```python
from build123d import *

# Parameters (mm, degrees)
F0_W     = 25
F0_H     = 31
F1_DEPTH = 86.3
F2_R     = 6.5
F3_DEPTH = 31.5
F5_DEPTH = 31.001


with BuildPart() as f1:
    # F0 (on Top) → F1 (new body)
    with BuildSketch(Plane.XY):
        Rectangle(F0_W, F0_H)
    extrude(amount=F1_DEPTH)

    # F2 (on Front) → F3 (cut, symmetric)
    with BuildSketch(Plane.XZ):
        with Locations((0, 58.577)):
            Circle(F2_R)
    extrude(amount=F3_DEPTH, both=True, mode=Mode.SUBTRACT)

    # F4 (on face) → F5 (cut, through all)
    with BuildSketch(Plane(origin=(0, 15.5, 0), x_dir=(-1, 0, 0), z_dir=(0, 1, 0))):
        Polygon((12.5, 0), (12.5, 86.3), (6, 0), align=None)
        Polygon((-6, 0), (-12.5, 86.3), (-12.5, 0), align=None)
    extrude(amount=-F5_DEPTH, mode=Mode.SUBTRACT)


solid = f1.part
```
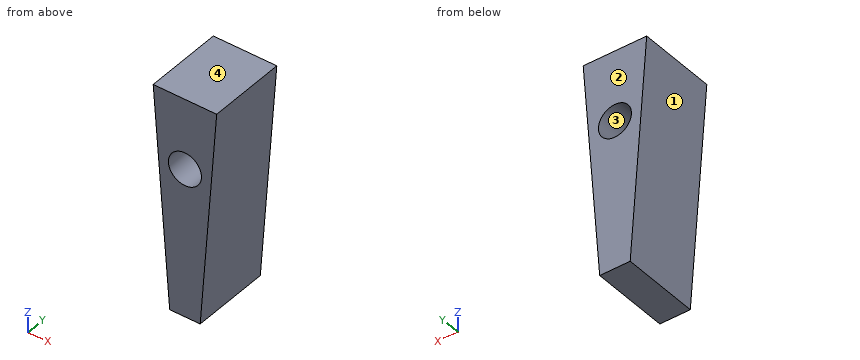
Check sheet for the modelled part. Datum: model origin and axes. Units: mm. Face numbers are marked on the shaded views. Round coordinates to 2 decimals unless told otherwise and drop trailing zeros. Order: outer loops, then holes, each group sorted by start corner. A loop starts at its lowest first (then second) coordinate and runs counter-clockwise, first axis right, second up.
1) Section check D-D (z = 31). Record the boundary of the cut face in (x, y), and give its area (3 significant figures).
2) Section check B-B (z = 60.5). Record the boundary of the cut face in (x, y).
3) Section check C-C (y = 1). Record the boundary of the cut face in (x, z).
4) Section check A-A (x = 0). Record the boundary of the cut face in (y, z).
5) Mould release check, pull along Z, two halves, no side actions. Record for the marked faces 1, 2, 3 and 4: +Z half, -Z half, draft (parallel to the pull), parting line (faces both ways), or undercut.
6) Scan lines: line 1 (Z direction, x = 0, y = -2); line 2 (X direction, y = 7.5, z = 63); line 3 (X direction, y = 7.5, z = 56.5). Record each from-to range of solid material in increasing order.
7) Go/stop test with flat-tipped pins: pin 1 Ø1 at (y, z) = (-12, 17) entering from -X; pin 2 Ø2 at (y, z) = (-9.5, 27) entering from +X; pin 3 Ø15 at (x, z) = (0, 58.577) entering from +Y; pin 4 Ø12 at (y, z) = (10.5, 63) entering from -X. Record where each tip stops, or that it passes through.
Result:
1. outline: (-8.33, -15.5) - (8.33, -15.5) - (8.33, 15.5) - (-8.33, 15.5) - close
1. area: 517 mm2
2. outline: (-10.56, -15.5) - (-6.21, -15.5) - (-6.21, 15.5) - (-10.56, 15.5) - close; (6.21, -15.5) - (10.56, -15.5) - (10.56, 15.5) - (6.21, 15.5) - close
3. outline: (-12.5, 86.3) - (-6, 0) - (6, 0) - (12.5, 86.3) - close; hole circle Ø13 at (0, 58.58)
4. outline: (-15.5, 0) - (15.5, 0) - (15.5, 52.08) - (-15.5, 52.08) - close; (-15.5, 65.08) - (15.5, 65.08) - (15.5, 86.3) - (-15.5, 86.3) - close
5. face 1: -Z half
5. face 2: draft
5. face 3: undercut
5. face 4: +Z half
6. line 1: z = 0 to 52.08, 65.08 to 86.3
6. line 2: x = -10.75 to -4.76, 4.76 to 10.75
6. line 3: x = -10.26 to -6.16, 6.16 to 10.26
7. pin 1: stops at x = -7.32
7. pin 2: stops at x = 8.11
7. pin 3: stops at y = 15.5
7. pin 4: stops at x = -11.2
